Design review of the part built by this model. Coordinates are the model's own, in mm. Face numbers are marked on the shaded views. A direction names the side the tool comes from. Give positions to 0.01 mm unless a question says otherwise; leave off trailing zeros. Order: outer loops, then holes, each group sorted by start corner. A loop starts at its lowest first (then second) coordinate and runs counter-clockwise, first axis right, second up. Notation, with made-up numbers: M 13,-15.5 L 57,-15.5 A11 ccw 57,-6.5 Z; hole C 79.25,51 d11. An arc over 180 degrees is marked long. Answer as a JSON object with one key per item and string values.
from build123d import *

# Parameters (mm, degrees)
F1_DEPTH    = 3
F2_DEPTH    = 11.9
F4_DEPTH    = 1
F6_DEPTH    = 6
F7_T1_DEPTH = 40.9
F8_R        = 2
F9_R        = 3.5272638361
F10_DEPTH   = 1
F11_DEPTH   = 1


# Not quite as in the source:
# - a fillet or chamfer that OpenCascade refuses, or shapes differently, is made with other operations: its cross-section is extruded or revolved along the edge and cut away or added


with BuildPart() as f1:
    # F0 (on Top) → F1 (new body)
    with BuildSketch(Plane.XY):
        with BuildLine():
            Line((13.35, -34.6), (13.35, 0))
            ThreePointArc((13.35, 0), (0, 13.35), (-13.35, 0))
            Line((-13.35, 0), (-13.35, -34.6))
            Line((-13.35, -34.6), (13.35, -34.6))
        make_face()
        with BuildLine():
            Line((-10.35, -31.6), (-10.35, 0))
            ThreePointArc((-10.35, 0), (0, 10.35), (10.35, 0))
            Line((10.35, 0), (10.35, -31.6))
            Line((10.35, -31.6), (-10.35, -31.6))
        make_face(mode=Mode.SUBTRACT)
        with BuildLine():
            ThreePointArc((10.35, 0), (0, 10.35), (-10.35, 0))
            Line((-10.35, 0), (-10.35, -31.6))
            Line((-10.35, -31.6), (10.35, -31.6))
            Line((10.35, -31.6), (10.35, 0))
        make_face()
    extrude(amount=-F1_DEPTH)

    # F0 (on Top) → F2 (join)
    with BuildSketch(Plane.XY):
        with BuildLine():
            Line((13.35, -34.6), (13.35, 0))
            ThreePointArc((13.35, 0), (0, 13.35), (-13.35, 0))
            Line((-13.35, 0), (-13.35, -34.6))
            Line((-13.35, -34.6), (13.35, -34.6))
        make_face()
        with BuildLine():
            Line((-10.35, -31.6), (-10.35, 0))
            ThreePointArc((-10.35, 0), (0, 10.35), (10.35, 0))
            Line((10.35, 0), (10.35, -31.6))
            Line((10.35, -31.6), (-10.35, -31.6))
        make_face(mode=Mode.SUBTRACT)
    extrude(amount=F2_DEPTH)

    # F3 (on face) → F4 (join)
    with BuildSketch(Plane.XY.offset(11.9)):
        Polygon((-13.35, -34.6), (13.35, -34.6), (13.35, -31.6), (10.35, -31.6), (-10.35, -31.6), (-13.35, -31.6), align=None)
    extrude(amount=F4_DEPTH)

    # F5 (on face) → F6 (cut)
    with BuildSketch(Plane.XZ.offset(34.6)):
        with BuildLine():
            ThreePointArc((0, 9.2), (-2.15, 7.05), (0, 4.9))
            Line((0, 4.9), (0, 9.2))
        make_face()
        with BuildLine():
            Line((0, 9.2), (0, 4.9))
            ThreePointArc((0, 4.9), (1.5202795796, 5.5297204204), (2.15, 7.05))
            ThreePointArc((2.15, 7.05), (1.5202795796, 8.5702795796), (0, 9.2))
        make_face()
    extrude(amount=-F6_DEPTH, mode=Mode.SUBTRACT)

    # F7: fillet of radius 5 on 2 edges, made by hand

    # F7_s2 → F7_t1 (cut)
    with BuildSketch(Plane.XY.offset(-15.5)):
        with BuildLine():
            ThreePointArc((-13.35, -29.6), (-11.8855339059, -33.1355339059), (-8.35, -34.6))
            Line((-8.35, -34.6), (-13.35, -34.6))
            Line((-13.35, -34.6), (-13.35, -29.6))
        make_face()
        with BuildLine():
            ThreePointArc((8.35, -34.6), (11.8855339059, -33.1355339059), (13.35, -29.6))
            Line((13.35, -29.6), (13.35, -34.6))
            Line((13.35, -34.6), (8.35, -34.6))
        make_face()
    extrude(amount=F7_T1_DEPTH, mode=Mode.SUBTRACT)

    # F8
    f8_edges = [f1.edges().sort_by_distance(p)[0] for p in [
        (13.35, -14.8, -3),
    ]]
    fillet(f8_edges, radius=F8_R)

    # F9 (on face) → F10 (join)
    with BuildSketch(Plane(origin=(0, -31.6, 0), x_dir=(-1, 0, 0), z_dir=(0, 1, 0))):
        with Locations((0, 7.05)):
            Circle(F9_R)
    extrude(amount=-F10_DEPTH)

    # F11 (add): a face of the model
    f11_faces = [f1.faces().sort_by_distance(p)[0] for p in [
        (0, -32.6, 7.05),
    ]]
    extrude(f11_faces, amount=F11_DEPTH)


solid = f1.part
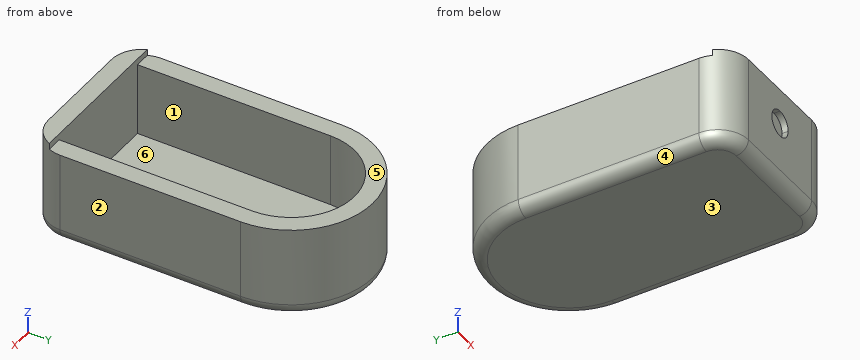
(1) We need section A-A (z = 11). Write out the cut boundary in (x, y).
Checked values:
{"outline": "M -13.35,-29.6 A5 ccw -8.35,-34.6 L 8.35,-34.6 A5 ccw 13.35,-29.6 L 13.35,0 A13.35 ccw -13.35,0 Z; hole M -10.35,-31.6 L 10.35,-31.6 L 10.35,0 A10.35 ccw -10.35,0 Z"}
(2) Draft analysis for pull direction X (two halves, no side actions). For the marked faces 1, 2 and 3, state which applies: +X half, -X half, draft (parallel to the pull), parting line (faces both ways), or undercut.
Checked values:
{"face 1": "undercut", "face 2": "+X half", "face 3": "draft"}
(3) We need section B-B (y = -15.5). Write out the cut boundary in (x, z), plus the area to 3 significant figures.
Checked values:
{"outline": "M -13.35,-1 A2 ccw -11.35,-3 L 11.35,-3 A2 ccw 13.35,-1 L 13.35,11.9 L 10.35,11.9 L 10.35,0 L -10.35,0 L -10.35,11.9 L -13.35,11.9 Z", "area": "150 mm^2"}
(4) Insertion check: pin 1 (5 mm diameter, centred on x = 3.5, z = 10.5, fed in from +Y); pin 2 (1.5 mm diameter, centred on x = -1, y = 3, fed in from +Z); pin 3 (1.3 mm diameter, centred on x = 0, z = 6.5, fed in from -Y). Each pin has a flat end and moves straight along its axis. Give the tip position at first contact, or say it passes through.
Checked values:
{"pin 1": "stops at y = 13.31", "pin 2": "stops at z = 0", "pin 3": "stops at y = -33.6"}
(5) Tool access review of the marked faces 4, 5 and 6: name each direction out of +Z, -Z, +X, -X, +Y, -Y from which nothing blocks a thin tool from reaching the whole face with its end or side.
Checked values:
{"face 4": "-Z, -X, +Y, -Y", "face 5": "+Z, +X, -X, +Y", "face 6": "+Z"}
(6) To check wall thickness, follow L1, parallel to X at y = -26, z = 4.75; L2, parallel to Z at x = 5, y = -27.5. State the ranges of each line that lie inside material, in increasing order. Write a range as from..to.
Checked values:
{"L1": "x = -13.35..-10.35, 10.35..13.35", "L2": "z = -3..0"}
